```python
from build123d import *

# Parameters (mm, degrees)
F0_R     = 3
F0_R_2   = 2.5
F1_DEPTH = 973
F2_R     = 2
F3_R     = 7
F5_DEPTH = 60


# Not quite as in the source:
# - a feature names something its author has since deleted; it is built from what else it names


with BuildPart() as f1:
    # F0 (on Top) → F1 (new body)
    with BuildSketch(Plane.XY):
        with BuildLine():
            Line((18.15, -30), (30, -30))
            Line((30, -30), (30, -18.15))
            Line((30, -18.15), (27.5, -18.15))
            Line((27.5, -18.15), (27.5, -20.15))
            Line((27.5, -20.15), (21.5477069044, -20.15))
            ThreePointArc((21.5477069044, -20.15), (19.5, -15), (21.5477069044, -9.85))
            Line((21.5477069044, -9.85), (27.5, -9.85))
            Line((27.5, -9.85), (27.5, -11.85))
            Line((27.5, -11.85), (30, -11.85))
            Line((30, -11.85), (30, 11.85))
            Line((30, 11.85), (27.5, 11.85))
            Line((27.5, 11.85), (27.5, 9.85))
            Line((27.5, 9.85), (21.5477069044, 9.85))
            ThreePointArc((21.5477069044, 9.85), (19.5, 15), (21.5477069044, 20.15))
            Line((21.5477069044, 20.15), (27.5, 20.15))
            Line((27.5, 20.15), (27.5, 18.15))
            Line((27.5, 18.15), (30, 18.15))
            Line((30, 18.15), (30, 30))
            Line((30, 30), (18.15, 30))
            Line((18.15, 30), (18.15, 27.5))
            Line((18.15, 27.5), (20.15, 27.5))
            Line((20.15, 27.5), (20.15, 21.5477069044))
            ThreePointArc((20.15, 21.5477069044), (15, 19.5), (9.85, 21.5477069044))
            Line((9.85, 21.5477069044), (9.85, 27.5))
            Line((9.85, 27.5), (11.85, 27.5))
            Line((11.85, 27.5), (11.85, 30))
            Line((11.85, 30), (-11.85, 30))
            Line((-11.85, 30), (-11.85, 27.5))
            Line((-11.85, 27.5), (-9.85, 27.5))
            Line((-9.85, 27.5), (-9.85, 21.5477069044))
            ThreePointArc((-9.85, 21.5477069044), (-15, 19.5), (-20.15, 21.5477069044))
            Line((-20.15, 21.5477069044), (-20.15, 27.5))
            Line((-20.15, 27.5), (-18.15, 27.5))
            Line((-18.15, 27.5), (-18.15, 30))
            Line((-18.15, 30), (-30, 30))
            Line((-30, 30), (-30, 18.15))
            Line((-30, 18.15), (-27.5, 18.15))
            Line((-27.5, 18.15), (-27.5, 20.15))
            Line((-27.5, 20.15), (-21.5477069044, 20.15))
            ThreePointArc((-21.5477069044, 20.15), (-19.5, 15), (-21.5477069044, 9.85))
            Line((-21.5477069044, 9.85), (-27.5, 9.85))
            Line((-27.5, 9.85), (-27.5, 11.85))
            Line((-27.5, 11.85), (-30, 11.85))
            Line((-30, 11.85), (-30, -11.85))
            Line((-30, -11.85), (-27.5, -11.85))
            Line((-27.5, -11.85), (-27.5, -9.85))
            Line((-27.5, -9.85), (-21.5477069044, -9.85))
            ThreePointArc((-21.5477069044, -9.85), (-19.5, -15), (-21.5477069044, -20.15))
            Line((-21.5477069044, -20.15), (-27.5, -20.15))
            Line((-27.5, -20.15), (-27.5, -18.15))
            Line((-27.5, -18.15), (-30, -18.15))
            Line((-30, -18.15), (-30, -30))
            Line((-30, -30), (-18.15, -30))
            Line((-18.15, -30), (-18.15, -27.5))
            Line((-18.15, -27.5), (-20.15, -27.5))
            Line((-20.15, -27.5), (-20.15, -21.5477069044))
            ThreePointArc((-20.15, -21.5477069044), (-15, -19.5), (-9.85, -21.5477069044))
            Line((-9.85, -21.5477069044), (-9.85, -27.5))
            Line((-9.85, -27.5), (-11.85, -27.5))
            Line((-11.85, -27.5), (-11.85, -30))
            Line((-11.85, -30), (11.85, -30))
            Line((11.85, -30), (11.85, -27.5))
            Line((11.85, -27.5), (9.85, -27.5))
            Line((9.85, -27.5), (9.85, -21.5477069044))
            ThreePointArc((9.85, -21.5477069044), (15, -19.5), (20.15, -21.5477069044))
            Line((20.15, -21.5477069044), (20.15, -27.5))
            Line((20.15, -27.5), (18.15, -27.5))
            Line((18.15, -27.5), (18.15, -30))
        make_face()
        with Locations((-25, -25)):
            Circle(F0_R, mode=Mode.SUBTRACT)
        with Locations((-15, -15)):
            Circle(F0_R_2, mode=Mode.SUBTRACT)
        with Locations((25, -25)):
            Circle(F0_R, mode=Mode.SUBTRACT)
        with Locations((15, -15)):
            Circle(F0_R_2, mode=Mode.SUBTRACT)
        with Locations((-25, 25)):
            Circle(F0_R, mode=Mode.SUBTRACT)
        with Locations((-15, 15)):
            Circle(F0_R_2, mode=Mode.SUBTRACT)
        Polygon((-7, 22), (-7, 27.5), (0, 27.5), (7, 27.5), (7, 22), (10, 16), (10, 10), (16, 10), (22, 7), (27.5, 7), (27.5, 0), (27.5, -7), (22, -7), (16, -10), (10, -10), (10, -16), (7, -22), (7, -27.5), (0, -27.5), (-7, -27.5), (-7, -22), (-10, -16), (-10, -10), (-16, -10), (-22, -7), (-27.5, -7), (-27.5, 0), (-27.5, 7), (-22, 7), (-16, 10), (-10, 10), (-10, 16), align=None, mode=Mode.SUBTRACT)
        with Locations((15, 15)):
            Circle(F0_R_2, mode=Mode.SUBTRACT)
        with Locations((25, 25)):
            Circle(F0_R, mode=Mode.SUBTRACT)
    extrude(amount=F1_DEPTH)

    # F2
    f2_edges = [f1.edges().sort_by_distance(p)[0] for p in [
        (-7, 27.5, 486.5),
        (7, 27.5, 486.5),
    ]]
    fillet(f2_edges, radius=F2_R)

    # F3
    f3_edges = [f1.edges().sort_by_distance(p)[0] for p in [
        (-10, 16, 486.5),
        (10, 16, 486.5),
    ]]
    fillet(f3_edges, radius=F3_R)

    # F4 (on face) → F5 (cut)
    with BuildSketch(Plane.XZ.offset(30)):
        Polygon((30, 0), (30, 60), (-30, 0), (-18.15, 0), align=None)
        Polygon((30, 913), (30, 973), (-18.15, 973), (-30, 973), align=None)
    extrude(amount=-F5_DEPTH, mode=Mode.SUBTRACT)


solid = f1.part
```
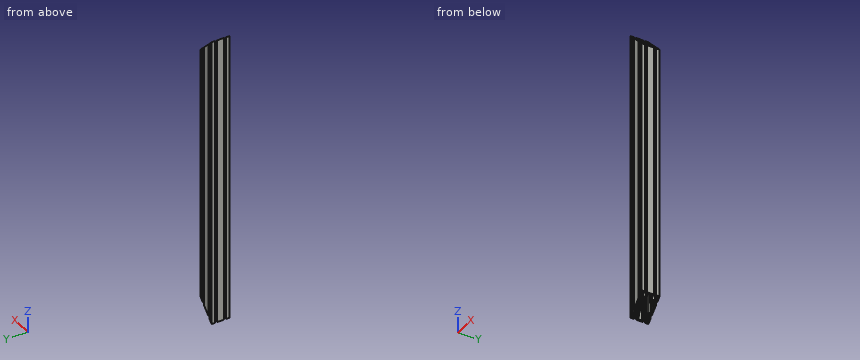
Input: part model. Units: mm. Frame: model coordinates. Give positions to 0.01 mm unless a question says otherwise; leave off trailing zeros. Answer as CSV lines item,"result". Start each with the question number.
1. Line query: L1, parallel to X at y = 28.5, z = 384; L2, parallel to Y at x = -25, z = 204; L3, parallel to Y at x = -15, z = 625. Output: solid intervals per line, ascending.
2. Section A-A on z = 594. State how many separate pieces and enclosed holes the cut face has, plus the area to 3 significant figures.
3. Pin query (flat end, axial travel): P1, Ø6, axis at x = -8, y = -23.5, coming from the -Z side; P2, Ø4, axis at x = -13.5, z = 713.5, coming from the -Y side; P3, Ø1, axis at x = -15, z = 330, coming from the +Y side; P4, Ø1.8, axis at x = 13, z = 514, coming from the +Y side. Return the tip coordinate at first contact, or that it passes through.
Computed values:
1,L1,"x = -30 to -18.15, -11.85 to 11.85, 18.15 to 30"
1,L2,"y = -30 to -28, -22 to -20.15, -9.85 to -7, 7 to 9.85, 20.15 to 22, 28 to 30"
1,L3,"y = -19.5 to -17.5, -12.5 to -10, 10 to 12.5, 17.5 to 19.5"
2,separate pieces,"1"
2,enclosed holes,"9"
2,area,"1,080 mm²"
3,P1,"stops at z = 19.92"
3,P2,"stops at y = -30"
3,P3,"stops at y = 19.52"
3,P4,"stops at y = 20.08"
